Here's how the part is built. I have some questions about the finished solid (model axes, mm). Face numbers are marked on the shaded views. Give positions to 0.01 mm unless a question says otherwise; leave off trailing zeros. Order: outer loops, then holes, each group sorted by start corner. A loop starts at its lowest first (then second) coordinate and runs counter-clockwise, first axis right, second up. Notation, with made-up numbers: M 27.5,48.5 L 78.5,48.5 A24 ccw 78.5,80.5 Z; hole C -22.5,88.25 d9. An arc over 180 degrees is marked long. One line per item, written item: value. Start each with the question number.
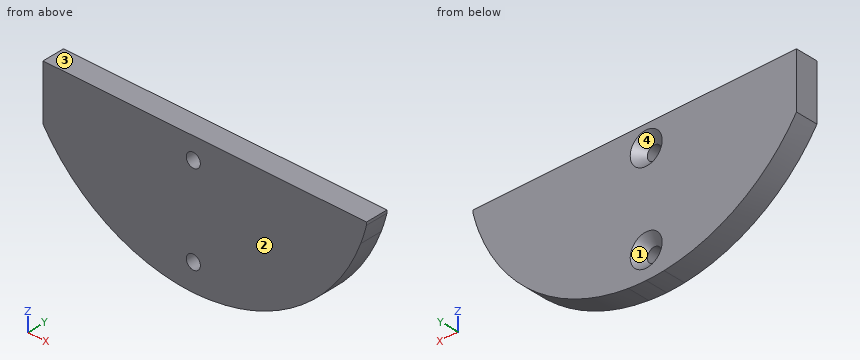
from build123d import *

# Parameters (mm, degrees)
SKETCH1_R           = 2
BOSS_EXTRUDE1_DEPTH = 6.35
CHAMFER1_SIZE       = 2.54


with BuildPart() as part:
    # Sketch1 → Boss-Extrude1 (new body)
    with BuildSketch(Plane(origin=(0, 0, 0), x_dir=(1, 0, 0), z_dir=(0, 1, 0))):
        with BuildLine():
            Line((-42.746, 11.684), (47.586884748, 11.684))
            Line((47.586884748, 11.684), (47.586884748, 17.78))
            ThreePointArc((47.586884748, 17.78), (31.011055518, 40.236232871), (5.073646026, 50.546))
            Line((5.073646026, 50.546), (-5.073646026, 50.546))
            ThreePointArc((-5.073646026, 50.546), (-26.552841725, 43.308043091), (-42.746, 27.448487827))
            Line((-42.746, 27.448487827), (-42.746, 11.684))
        make_face()
        with Locations((0, 17.78)):
            Circle(SKETCH1_R, mode=Mode.SUBTRACT)
        with Locations((0, 43.18)):
            Circle(SKETCH1_R, mode=Mode.SUBTRACT)
        with BuildLine():
            Line((47.586884748, 17.78), (47.586884748, 11.684))
            Line((47.586884748, 11.684), (49.243425186, 11.684))
            Line((49.243425186, 11.684), (49.243425186, 12.478985375))
            ThreePointArc((49.243425186, 12.478985375), (48.487652237, 15.15214772), (47.586884748, 17.78))
        make_face()
        with BuildLine():
            Line((-5.073646026, 50.546), (5.073646026, 50.546))
            ThreePointArc((5.073646026, 50.546), (2.539999948, 50.736460265), (-1.05e-07, 50.8))
            ThreePointArc((-1.05e-07, 50.8), (-2.540000052, 50.73646026), (-5.073646026, 50.546))
        make_face()
    extrude(amount=BOSS_EXTRUDE1_DEPTH)

    # Chamfer1
    chamfer1_edges = [part.edges().sort_by_distance(p)[0] for p in [
        (-2, 6.35, -17.78),
        (-2, 6.35, -43.18),
    ]]
    chamfer(chamfer1_edges, length=CHAMFER1_SIZE)


solid = part.part
Item 1: I want a section at A-A on y = 3. Write out the boundary of the cut face in (x, z).
Item 2: We'd pull the mould along Z, two halves only. Please class the marked faces 1, 2, 3 and 4: +Z half, -Z half, draft (parallel to the pull), parting line (faces both ways), or undercut.
Item 3: Please list where these lines run through material, in increasing order: probe 1 along Z at (x, y) = (0, 3); probe 2 along Z at (x, y) = (1.5, 3.25); probe 3 along X at (y, z) = (1.8, -17.78). Write a range as [from, to].
Item 4: I want a section at C-C on x = 12.5. Write out the boundary of the cut face in (y, z), plus the area to 3 significant figures.
Item 5: I want a section at D-D on z = -35. Write out the boundary of the cut face in (x, y).
Item 6: I want a section at B-B on z = -43.18. Write out the boundary of the cut face in (x, y), plus the area to 3 significant figures.
Item 7: Will these pins go through, and if not, where does the flat tip stop? P1, Ø3, axis at y = 1, z = -19, coming from the +X side; P2, Ø2, axis at x = 9, z = -30.5, coming from the -Y side; P3, Ø2.5, axis at x = 0, z = -17.78, coming from the +Y side; P4, Ø1, axis at y = 3, z = -33, coming from the +X side.
Answer below:
1. outline: M -42.75,-27.45 A50.8 ccw 49.24,-12.48 L 49.24,-11.68 L -42.75,-11.68 Z; hole C 0,-43.18 d4; hole C 0,-17.78 d4
2. face 1: undercut
2. face 2: draft
2. face 3: +Z half
2. face 4: undercut
3. probe 1: z = [-50.8, -45.18], [-41.18, -19.78], [-15.78, -11.68]
3. probe 2: z = [-50.78, -44.5], [-41.86, -19.1], [-16.46, -11.68]
3. probe 3: x = [-42.75, -2], [2, 47.59]
4. outline: M 0,-49.24 L 6.35,-49.24 L 6.35,-11.68 L 0,-11.68 Z
4. area: 238 mm²
5. outline: M -36.82,0 L 36.82,0 L 36.82,6.35 L -36.82,6.35 Z
6. outline: M -26.76,0 L -2,0 L -2,3.81 L -4.54,6.35 L -26.76,6.35 Z; M 2,0 L 26.76,0 L 26.76,6.35 L 4.54,6.35 L 2,3.81 Z
6. area: 308 mm²
7. P1: stops at x = 47.69
7. P2: stops at y = 0
7. P3: passes through
7. P4: stops at x = 39.04
